Geometry check sheet. Reference: the model listing, model coordinates, mm. A direction names the side the tool comes from. Round coordinates to 2 decimals unless told otherwise and drop trailing zeros. Order: outer loops, then holes, each group sorted by start corner. A loop starts at its lowest first (then second) coordinate and runs counter-clockwise, first axis right, second up. Notation, with made-up numbers: (-15.75, 46) - (-1.75, 46) arc R14 cw to (-1.75, 67) - close; hole circle Ø3 at (1, 45.5). An arc over 180 degrees is marked (long way). Write each question's results on one line, items separated by ' | '.
Autodesk Inventor part; units mm, degrees
ref_plane "Start Plane" through (0, 0, 0) normal (0, 0, 1) x (1, 0, 0)
ref_plane "End Plane" through (0, 0, 260) normal (0, 0, 1) x (1, 0, 0)
ref_plane "Work Plane6" through (0, 1060, 0) normal (0.3846, 0, -0.9231) x (-0.9231, 0, -0.3846)
ref_plane "Start Plane" through (0, 0, 0) normal (0, 0, 1) x (1, 0, 0)
ref_plane "End Plane" through (0, 0, 260) normal (0, 0, 1) x (1, 0, 0)
sketch "Sketch" plane through (0, 0, 0) normal (0, 0, 1) x (1, 0, 0)
  line L0 (25.4, 0) -> (0, 0)
  line L1 (0, 0) -> (0, 25.4)
  line L2 (0, 25.4) -> (1.651, 25.4)
  line L3 (3.175, 23.876) -> (3.175, 6.477)
  line L4 (6.477, 3.175) -> (23.876, 3.175)
  line L5 (25.4, 1.651) -> (25.4, 0)
  line L6 (0, -11.0414) -> (0, 31.5385) construction
  line L7 (-11.0414, 0) -> (31.5385, 0) construction
  arc A0 (3.175, 6.477) -> (6.477, 3.175) centre (6.477, 6.477) ccw
  arc A1 (3.175, 23.876) -> (1.651, 25.4) centre (1.651, 23.876) ccw
  arc A2 (25.4, 1.651) -> (23.876, 3.175) centre (23.876, 1.651) ccw
  line L8 (0, 40.0545) -> (0, -19.5574) construction
  line L9 (-19.5574, 0) -> (40.0545, 0) construction
  point P0 (3.175, 25.4)
  point P1 (3.175, 3.175)
  point P2 (25.4, 3.175)
  dimension "d0" = 25.4
  dimension "d1" = 25.4
  dimension "d2" = 3.175
  dimension "d3" = 3.175
  dimension "d10" = 0
  dimension "d11" = 0
  dimension "d14" = 3.302
  dimension "d15" = 1.524
extrude "Body" add sketch "Sketch" along normal up to surface (260 mm away) from surface at 0
sketch "Sketch3" plane through (0, 0, 0) normal (0, 0, 1) x (1, 0, 0)
  line L0 (0, 0) -> (10, 0)
ref_plane "Work Plane3" through (0, 0, 0) normal (0, -1, 0) x (1, 0, 0)
ref_plane "Work Plane6" through (0, 1060, 0) normal (0.3846, 0, -0.9231) x (-0.9231, 0, -0.3846)
split "Split3" plane through (0, 1060, 0) removes the side toward (0.3846, 0, -0.9231)
sketch "Sketch4" plane through (0, 0, 0) normal (0, -1, 0) x (1, 0, 0)
  line L0 (-2, 0) -> (12, 0)
  line L1 (-2, 260) -> (12, 260)
  dimension "d17" = 260
equation "\"d0\" = G_H"
equation "\"d1\" = G_H"
equation "\"d2\" = G_T"
equation "\"d3\" = G_T"
equation "\"d14\" = G_IR"
equation "\"d15\" = G_ER"
equation "\"d4\" = G_L"
equation "\"G_H\" = 25.4"
equation "\"G_T\" = 3.175"
equation "\"G_ER\" = 1.524"
equation "\"G_IR\" = 3.302"
equation "\"G_L\" = d17"
equation "\"ex\" = 0"
equation "\"G_OFFSET_START\" = 0"
equation "\"G_OFFSET_END\" = 0"
equation "\"d13\" = G_OFFSET_END + B_L"
equation "\"B_L\" = 260"
properties part number "AISC - L 1 x 1 x 1/8 - 10.236" material "Steel, Mild"
(1) Depth check by flat-ended pin: pin 1 Ø2 at (x, y) = (3, 11) entering from -Z; pin 2 Ø3 at (x, y) = (6, 4) entering from -Z; pin 3 Ø14 at (y, z) = (13, 69) entering from +X. Enter the tip coordinate at first touch or a pass-through.
Answers follow:
pin 1: z = 0.83 | pin 2: z = 1.88 | pin 3: x = 3.21
(2) Material ranges on line 1 (X direction, y = 8.75, z = 111) (3 decimals); line 2 (X direction, y = 1.75, z = 185), recorded low to high.
Answers follow:
line 1: 0 to 3.175 | line 2: 0 to 25.4
(3) Access from +Z, -Z, +X, -X, +Y, -Y to the whole of each face (thin tool, end or side, straight path). Record for faces 1 (the face through (3.175, 15, 129)), 2 (the face through (13, 0, 128)).
Answers follow:
face 1: +Z, -Z, +X, +Y | face 2: +Z, -Z, +X, -X, -Y
(4) Section check A-A (z = 72). Record the cut outline in (x, y) (3 decimals), then the cut area to 3 significant figures.
Answers follow:
outline: (0, 0) - (25.4, 0) - (25.4, 1.651) arc R1.524 ccw to (23.876, 3.175) - (6.477, 3.175) arc R3.302 cw to (3.175, 6.477) - (3.175, 23.876) arc R1.524 ccw to (1.651, 25.4) - (0, 25.4) - close | area: 153 mm²
(5) Section check C-C (x = 12.25). Record the cut outline in (y, z) (3 decimals), then the cut area to 3 significant figures.
Answers follow:
outline: (0, 5.104) - (3.175, 5.104) - (3.175, 260) - (0, 260) - close | area: 809 mm²
(6) Section check B-B (y = 16.5). Record the cut outline in (x, z) (3 decimals), then the cut area to 3 significant figures.
Answers follow:
outline: (0, 0) - (3.175, 1.323) - (3.175, 260) - (0, 260) - close | area: 823 mm²
